from build123d import *

# Parameters (mm, degrees)
SKETCH1_W           = 300
SKETCH1_H           = 300
BOSS_EXTRUDE1_DEPTH = 6.35
CUT_EXTRUDE1_DEPTH  = 6.35
CUT_EXTRUDE2_DEPTH  = 425.311586573
SKETCH4_R           = 3.5
CUT_EXTRUDE3_DEPTH  = 10


with BuildPart() as part:
    # Sketch1 → Boss-Extrude1 (new body)
    with BuildSketch(Plane.XY):
        with Locations((150, 150)):
            Rectangle(SKETCH1_W, SKETCH1_H)
    extrude(amount=BOSS_EXTRUDE1_DEPTH)

    # Sketch2 → Cut-Extrude1 (cut)
    with BuildSketch(Plane.XY.offset(6.35)):
        with BuildLine():
            Line((143.65, 210), (143.65, 260))
            ThreePointArc((143.65, 260), (150, 266.35), (156.35, 260))
            Line((156.35, 260), (156.35, 210))
            ThreePointArc((156.35, 210), (150, 203.65), (143.65, 210))
        make_face()
        with BuildLine():
            Line((181.35, 210), (181.35, 260))
            ThreePointArc((181.35, 260), (175, 266.35), (168.65, 260))
            Line((168.65, 260), (168.65, 210))
            ThreePointArc((168.65, 210), (175, 203.65), (181.35, 210))
        make_face()
        with BuildLine():
            Line((206.35, 210), (206.35, 260))
            ThreePointArc((206.35, 260), (200, 266.35), (193.65, 260))
            Line((193.65, 260), (193.65, 210))
            ThreePointArc((193.65, 210), (200, 203.65), (206.35, 210))
        make_face()
        with BuildLine():
            Line((231.35, 210), (231.35, 260))
            ThreePointArc((231.35, 260), (225, 266.35), (218.65, 260))
            Line((218.65, 260), (218.65, 210))
            ThreePointArc((218.65, 210), (225, 203.65), (231.35, 210))
        make_face()
        with BuildLine():
            Line((256.35, 210), (256.35, 260))
            ThreePointArc((256.35, 260), (250, 266.35), (243.65, 260))
            Line((243.65, 260), (243.65, 210))
            ThreePointArc((243.65, 210), (250, 203.65), (256.35, 210))
        make_face()
        with BuildLine():
            Line((131.35, 210), (131.35, 260))
            ThreePointArc((131.35, 260), (125, 266.35), (118.65, 260))
            Line((118.65, 260), (118.65, 210))
            ThreePointArc((118.65, 210), (125, 203.65), (131.35, 210))
        make_face()
        with BuildLine():
            Line((106.35, 210), (106.35, 260))
            ThreePointArc((106.35, 260), (100, 266.35), (93.65, 260))
            Line((93.65, 260), (93.65, 210))
            ThreePointArc((93.65, 210), (100, 203.65), (106.35, 210))
        make_face()
        with BuildLine():
            Line((81.35, 210), (81.35, 260))
            ThreePointArc((81.35, 260), (75, 266.35), (68.65, 260))
            Line((68.65, 260), (68.65, 210))
            ThreePointArc((68.65, 210), (75, 203.65), (81.35, 210))
        make_face()
        with BuildLine():
            Line((56.35, 210), (56.35, 260))
            ThreePointArc((56.35, 260), (50, 266.35), (43.65, 260))
            Line((43.65, 260), (43.65, 210))
            ThreePointArc((43.65, 210), (50, 203.65), (56.35, 210))
        make_face()
    extrude(amount=-CUT_EXTRUDE1_DEPTH, mode=Mode.SUBTRACT)

    # Sketch3 → Cut-Extrude2 (cut, through all)
    with BuildSketch(Plane.XY.offset(6.35)):
        with BuildLine():
            Line((50, 80), (112.708755261, 80))
            ThreePointArc((112.708755261, 80), (132.708755261, 60), (112.708755261, 40))
            Line((112.708755261, 40), (50, 40))
            ThreePointArc((50, 40), (30, 60), (50, 80))
        make_face()
        with BuildLine():
            Line((250, 40), (187.708755261, 40))
            ThreePointArc((187.708755261, 40), (167.708755261, 60), (187.708755261, 80))
            Line((187.708755261, 80), (250, 80))
            ThreePointArc((250, 80), (270, 60), (250, 40))
        make_face()
    extrude(amount=-CUT_EXTRUDE2_DEPTH, mode=Mode.SUBTRACT)

    # Sketch4 → Cut-Extrude3 (cut)
    with BuildSketch(Plane.XY.offset(6.35)):
        with Locations((50, 287.5)):
            Circle(SKETCH4_R)
        with Locations((250, 287.5)):
            Circle(SKETCH4_R)
        with Locations((12.5, 50)):
            Circle(SKETCH4_R)
        with Locations((12.5, 250)):
            Circle(SKETCH4_R)
        with Locations(Location((287.5, 50, 0), (0, 0, 180))):
            Circle(SKETCH4_R)
        with Locations(Location((287.5, 250, 0), (0, 0, 180))):
            Circle(SKETCH4_R)
        with Locations(Location((250, 12.5, 0), (0, 0, 180))):
            Circle(SKETCH4_R)
        with Locations(Location((50, 12.5, 0), (0, 0, 180))):
            Circle(SKETCH4_R)
    extrude(amount=-CUT_EXTRUDE3_DEPTH, mode=Mode.SUBTRACT)


solid = part.part
Here's how the part is built. I have some questions about the finished solid (model axes, mm). A direction names the side the tool comes from. Give positions to 0.01 mm unless a question says otherwise; leave off trailing zeros. Loops run counter-clockwise (first coordinate to the right, second up) from the corner with the lowest first, then second, coordinate; pieces in that order, holes last. Notation, with made-up numbers: (48.25, -2.75) -> (64.25, -2.75) arc R23 cw to (64.25, 18.25) -> close; hole circle Ø8 at (41, 63). An arc over 180 degrees is marked (long way). Answer as a JSON object with one key per item and string values. Group by question number.
Item 1: I need wall thicknesses on L1, parallel to Y at x = 225.5, z = 0.75; L2, parallel to X at y = 12.5, z = 3. Which ranges of each line are inside material? Lowest first, please.
Item 2: Thinking about a two-plate mould opening in X: for faces 3 (the cylindrical face through (30, 60, 3)), 4 (the flat face through (148, 152, 0)), which applies, pulls with the +X half, pulls with the -X half, needs draft (parallel to the pull), parting line crosses it, or undercut?
Item 3: Imagine slicing it at B-B on x = 100. Write out the boundary of the cut face in (y, z).
Item 4: On a 3-axis mill with a long thin cutter (end or side, diameter ignored), from which of +Z, -Z, +X, -X, +Y, -Y can I reach the whole of each face in a straight line? I mean faces 1 (the cylindrical face through (167.714, 59.56, 3.219)), 2 (the flat face through (148, 152, 6.35)). Say none if no direction works.
Item 5: Imagine slicing it at C-C on x = 150. Write out the boundary of the cut face in (y, z), then the cut area to 3 significant figures.
Item 6: Imagine slicing it at D-D on y = 232. Give the number of separate pieces and of enclosed holes in the cut face, then the cut area to 3 significant figures.
Item 7: Imagine slicing it at A-A on y = 12.5. Write out the boundary of the cut face in (x, z), then the cut area to 3 significant figures.
Item 8: Will this pin go through, and if not, where does the flat tip stop? pin 1 (6.5 mm diameter, centred on x = 12.5, y = 50, fed in from -Z).
Answer list:
{
 "1": {"L1": "y = 0 to 40, 80 to 203.67, 266.33 to 300", "L2": "x = 0 to 46.5, 53.5 to 246.5, 253.5 to 300"},
 "2": {"face 3": "undercut", "face 4": "needs draft"},
 "3": {"outline": "(0, 0) -> (40, 0) -> (40, 6.35) -> (0, 6.35) -> close; (80, 0) -> (203.65, 0) -> (203.65, 6.35) -> (80, 6.35) -> close; (266.35, 0) -> (300, 0) -> (300, 6.35) -> (266.35, 6.35) -> close"},
 "4": {"face 1": "+Z, -Z", "face 2": "+Z, +X, -X, +Y, -Y"},
 "5": {"outline": "(0, 0) -> (203.65, 0) -> (203.65, 6.35) -> (0, 6.35) -> close; (266.35, 0) -> (300, 0) -> (300, 6.35) -> (266.35, 6.35) -> close", "area": "1,510 mm2"},
 "6": {"separate pieces": "10", "enclosed holes": "0", "area": "1,180 mm2"},
 "7": {"outline": "(0, 0) -> (46.5, 0) -> (46.5, 6.35) -> (0, 6.35) -> close; (53.5, 0) -> (246.5, 0) -> (246.5, 6.35) -> (53.5, 6.35) -> close; (253.5, 0) -> (300, 0) -> (300, 6.35) -> (253.5, 6.35) -> close", "area": "1,820 mm2"},
 "8": {"pin 1": "passes through"}
}
